Read the model definition and answer for the solid it produces. Units are mm, in the model's axes. Face numbers are marked on the shaded views. Coordinates: 2 decimals unless noted, no trailing zeros. Write each loop counter-clockwise with the first axis right and the second up, starting at its lowest first coordinate (ties: lowest second). Pieces come first, ordered by that corner, then holes. Notation, with made-up numbers: (-21.75, 68) -> (-3.75, 68) arc R11 cw to (-3.75, 77) -> close; hole circle Ø7 at (55.25, 35.25). An arc over 180 degrees is marked (long way). Write item = value, one per line. Start each with the question number.
1) Section A-A (x = 0) is taken. Determine the outline of the cut face in (y, z).
2) Section D-D (x = -135) is taken. Determine the outline of the cut face in (y, z), plus the area to 3 significant figures.
3) Section C-C (z = 32) is taken. Determine the outline of the cut face in (x, y).
4) A flat-ended cylindrical pin translates along its axis: pin 1 Ø10.5 at (x, y) = (-135, 0) entering from -Z. Find the tip coordinate at first contact, or state that the pin passes through.
5) Section B-B (y = 0) is taken. Determine the outline of the cut face in (x, z), plus the area to 3 significant figures.
6) Find the intervals of material crossed by line 1 along Y through (x, z) = (135, 21); line 2 along Y through (x, z) = (0, 8); line 3 along X through (y, z) = (-2.75, 14), in increasing order. Write a range as from..to.
7) For a pull along Y with two mould halves and no side action, classify the marked faces 1, 2 and 3 as released by +Y, released by -Y, zero draft, split by the parting line, or undercut.
from build123d import *

# Parameters (mm, degrees)
SKETCH1_W           = 300
SKETCH1_H           = 25
BOSS_EXTRUDE1_DEPTH = 35
SKETCH2_R           = 4.542391588
SKETCH2_R_2         = 11
CUT_EXTRUDE1_DEPTH  = 36


with BuildPart() as part:
    # Sketch1 → Boss-Extrude1 (new body)
    with BuildSketch(Plane.XY):
        Rectangle(SKETCH1_W, SKETCH1_H)
    extrude(amount=BOSS_EXTRUDE1_DEPTH)

    # Sketch2 → Cut-Extrude1 (cut, through all)
    with BuildSketch(Plane.XY.offset(35)):
        with Locations((-135, 0)):
            Circle(SKETCH2_R)
        Circle(SKETCH2_R_2)
        with Locations((135, 0)):
            Circle(SKETCH2_R)
    extrude(amount=-CUT_EXTRUDE1_DEPTH, mode=Mode.SUBTRACT)


solid = part.part
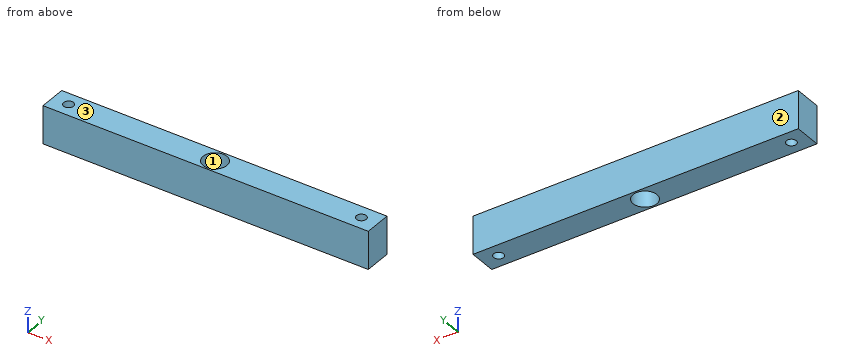
Answer key:
q1.outline = (-12.5, 0) -> (-11, 0) -> (-11, 35) -> (-12.5, 35) -> close; (11, 0) -> (12.5, 0) -> (12.5, 35) -> (11, 35) -> close
q2.outline = (-12.5, 0) -> (-4.54, 0) -> (-4.54, 35) -> (-12.5, 35) -> close; (4.54, 0) -> (12.5, 0) -> (12.5, 35) -> (4.54, 35) -> close
q2.area = 557 mm^2
q3.outline = (-150, -12.5) -> (150, -12.5) -> (150, 12.5) -> (-150, 12.5) -> close; hole circle Ø9.08 at (-135, 0); hole circle Ø22 at (0, 0); hole circle Ø9.08 at (135, 0)
q4.pin_1 = 0
q5.outline = (-150, 0) -> (-139.54, 0) -> (-139.54, 35) -> (-150, 35) -> close; (-130.46, 0) -> (-11, 0) -> (-11, 35) -> (-130.46, 35) -> close; (11, 0) -> (130.46, 0) -> (130.46, 35) -> (11, 35) -> close; (139.54, 0) -> (150, 0) -> (150, 35) -> (139.54, 35) -> close
q5.area = 9,090 mm^2
q6.line_1 = -12.5..-4.54, 4.54..12.5
q6.line_2 = -12.5..-11, 11..12.5
q6.line_3 = -150..-138.62, -131.38..-10.65, 10.65..131.38, 138.62..150
q7.face_1 = undercut
q7.face_2 = released by +Y
q7.face_3 = zero draft
